Here's how the part is built. I have some questions about the finished solid (model axes, mm). A direction names the side the tool comes from. Coordinates: 2 decimals unless noted, no trailing zeros. Write each loop counter-clockwise with the first axis right and the second up, starting at its lowest first coordinate (ties: lowest second). Pieces come first, ordered by that corner, then holes. Notation, with made-up numbers: M -15.5,-22 L 26.5,-22 A17 cw 26.5,0 Z; hole C -30.75,28.25 d8. An arc over 180 degrees is marked long. Write each question's results on one line, items separated by ' | '. Start each with the question number.
Autodesk Inventor part; units mm, degrees
ref_plane "Start plane" through (0, 0, 30) normal (0, 0, 1) x (1, 0, 0)
ref_plane "End plane" through (0, 0, 621) normal (0, 0, 1) x (1, 0, 0)
ref_plane "Work Plane5" through (1238.8, 45, 30) normal (0, 0, -1) x (-1, 0, 0)
ref_plane "Start plane" through (0, 0, 30) normal (0, 0, 1) x (1, 0, 0)
ref_plane "End plane" through (0, 0, 621) normal (0, 0, 1) x (1, 0, 0)
sketch "Sketch" plane through (0, 0, 0) normal (0, 0, 1) x (1, 0, 0)
  line L0 (-15, -11.25) -> (-15, 11.25)
  line L1 (-11.25, 15) -> (11.25, 15)
  line L2 (15, 11.25) -> (15, -11.25)
  line L3 (11.25, -15) -> (-11.25, -15)
  arc A0 (-15, -11.25) -> (-11.25, -15) centre (-11.25, -11.25) ccw
  arc A1 (-11.25, 15) -> (-15, 11.25) centre (-11.25, 11.25) ccw
  arc A2 (15, 11.25) -> (11.25, 15) centre (11.25, 11.25) ccw
  arc A3 (11.25, -15) -> (15, -11.25) centre (11.25, -11.25) ccw
  arc A4 (-11.25, 12.5) -> (-12.5, 11.25) centre (-11.25, 11.25) ccw
  line L4 (-11.25, 12.5) -> (11.25, 12.5)
  arc A5 (12.5, 11.25) -> (11.25, 12.5) centre (11.25, 11.25) ccw
  line L5 (12.5, 11.25) -> (12.5, -11.25)
  arc A6 (11.25, -12.5) -> (12.5, -11.25) centre (11.25, -11.25) ccw
  line L6 (11.25, -12.5) -> (-11.25, -12.5)
  arc A7 (-12.5, -11.25) -> (-11.25, -12.5) centre (-11.25, -11.25) ccw
  line L7 (-12.5, -11.25) -> (-12.5, 11.25)
  line L8 (0, 22.0873) -> (0, -22.0873) construction
  line L9 (-22.0873, 0) -> (22.0873, 0) construction
  dimension "d7" = 3.75
  dimension "d10" = 30
  dimension "d11" = 30
  dimension "d12" = 2.5
  dimension "d15" = 15
  dimension "d16" = 15
extrude "Body" add sketch "Sketch" along normal up to surface (591 mm away) from surface at 30
sketch "Sketch3" plane through (0, 0, 0) normal (0, 0, 1) x (1, 0, 0)
  line L0 (0, 0) -> (10, 0)
ref_plane "Work Plane3" through (0, 0, 0) normal (0, -1, 0) x (1, 0, 0)
sketch "Sketch4" plane through (0, 0, 0) normal (0, -1, 0) x (1, 0, 0)
  line L0 (-2, 30) -> (12, 30)
  line L1 (-2, 621) -> (12, 621)
  dimension "d18" = 591
ref_plane "Work Plane5" through (1238.8, 45, 30) normal (0, 0, -1) x (-1, 0, 0)
split "Split2" plane through (1238.8, 45, 30) removes the side toward (0, 0, -1)
ref_plane "Work Plane6" through (1297, -11.25, 621) normal (0, 0, 1) x (1, 0, 0)
split "Split3" plane through (1297, -11.25, 621) removes the side toward (0, 0, 1)
equation "\"d7\" = G_IR"
equation "\"d10\" = G_H"
equation "\"d11\" = G_W"
equation "\"d12\" = G_T"
equation "\"d15\" = 0.5 * d10"
equation "\"d16\" = 0.5 * d11"
equation "\"d3\" = G_L"
equation "\"G_W\" = 30"
equation "\"G_H\" = 30"
equation "\"G_T\" = 2.5"
equation "\"G_IR\" = 3.75"
equation "\"G_L\" = d18"
equation "\"d14\" = G_OFFSET_END + B_L"
equation "\"B_L\" = 651"
properties part number "DIN EN 10305-5 - 30 x 30 x 2,5  - 591" material "Steel, Mild"
1) For faces 1 (the flat face through (12.5, 0, 321)), 2 (the flat face through (-15, 0, 321)), which set-ups out of +Z, -Z, +X, -X, +Y, -Y let a thin tool reach every point of the face, with its end or its side?
2) We'd pull the mould along X, two halves only. Please class faces 3 (the flat face through (0, 12.5, 321)), 4 (the flat face through (15, 0, 321)), 5 (the flat face through (0, 15, 321)): pulls with the +X half, pulls with the -X half, needs draft (parallel to the pull), parting line crosses it, or undercut.
3) I want a section at A-A, the plane x = -2. Write out the boundary of the cut face in (y, z), then the cut area to 4 significant figures.
4) I want a section at B-B, the plane z = 464.5. Write out the boundary of the cut face in (x, y).
5) For pin 1 Ø12 at (x, y) = (5.5, 2.5) entering from +Z, with a flat end and sliding along its axis, tell me the tip position at first contact or that it passes through.
6) Please list where these lines run through material, in increasing order: line 1 (X direction, y = -1, z = 181); line 2 (X direction, y = 11.75, z = 275). Write a range as [from, to].
Output:
1) face 1: +Z, -Z | face 2: +Z, -Z, -X, +Y, -Y
2) face 3: undercut | face 4: pulls with the +X half | face 5: needs draft
3) outline: M -15,30 L -12.5,30 L -12.5,621 L -15,621 Z; M 12.5,30 L 15,30 L 15,621 L 12.5,621 Z | area: 2,955 mm2
4) outline: M -15,-11.25 A3.75 ccw -11.25,-15 L 11.25,-15 A3.75 ccw 15,-11.25 L 15,11.25 A3.75 ccw 11.25,15 L -11.25,15 A3.75 ccw -15,11.25 Z; hole M -12.5,-11.25 A1.25 ccw -11.25,-12.5 L 11.25,-12.5 A1.25 ccw 12.5,-11.25 L 12.5,11.25 A1.25 ccw 11.25,12.5 L -11.25,12.5 A1.25 ccw -12.5,11.25 Z
5) pin 1: passes through
6) line 1: x = [-15, -12.5], [12.5, 15] | line 2: x = [-14.97, -12.4], [12.4, 14.97]
